Answer from the drawing. Dimensions are ordinates in mm from the lowest x, y and z of the part. A direction names the side the tool comes from. Give positions to 0.01 mm unless a question says otherwise; leave off trailing zeros. Write each loop counter-clockwise with the first axis right and the second up, starting at its lowest first coordinate (ties: lowest second). Pieces come first, ordered by that corner, then holes.
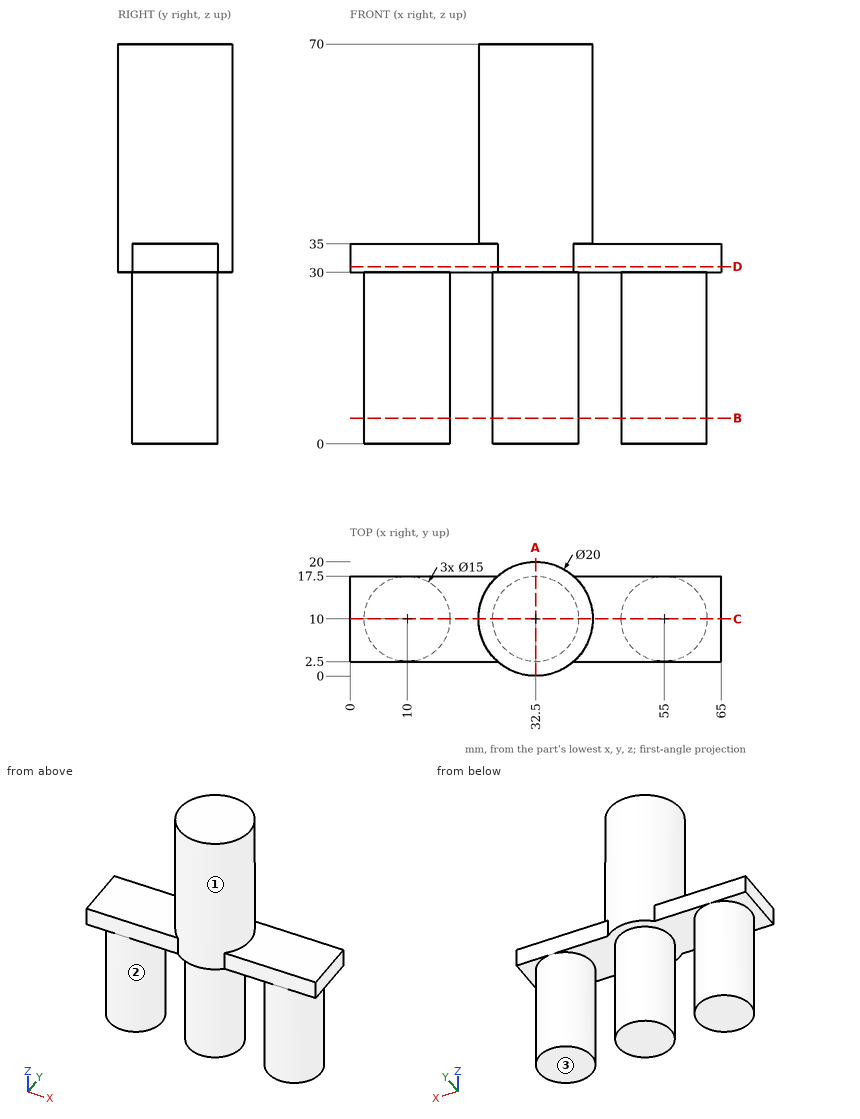
Item 1: A cutting plane is placed at C-C, the plane y = 10. Give the vertices of the cut face in (x, z).
Conclusion:
outline: (0, 30) - (2.5, 30) - (2.5, 0) - (17.5, 0) - (17.5, 30) - (25, 30) - (25, 0) - (40, 0) - (40, 30) - (47.5, 30) - (47.5, 0) - (62.5, 0) - (62.5, 30) - (65, 30) - (65, 35) - (42.5, 35) - (42.5, 70) - (22.5, 70) - (22.5, 35) - (0, 35) - close
Item 2: Each of these flat-tipped pins is pushed along its axis until it touches: P1, Ø5, axis at x = 9.5, y = 10, coming from the +Z side; P2, Ø8, axis at y = 11.5, z = 12, coming from the -X side; P3, Ø3, axis at x = 36, z = 38, coming from the +Y side. Where does it stop, or does it pass through?
Conclusion:
P1: stops at z = 35
P2: stops at x = 2.5
P3: stops at y = 19.8
Item 3: Which of the six approach directions +Z, -Z, +X, -X, +Y, -Y give full straight-line access (tool end or side, diameter ignored) to the marked faces 1, 2 and 3?
Conclusion:
face 1: +Z
face 2: -Z
face 3: -Z, +X, -X, +Y, -Y
Item 4: A cutting plane is placed at A-A, the plane x = 32.5. Give the vertices of the cut face in (y, z), plus the area to 3 significant figures.
Conclusion:
outline: (0, 30) - (2.5, 30) - (2.5, 0) - (17.5, 0) - (17.5, 30) - (20, 30) - (20, 70) - (0, 70) - close
area: 1,250 mm2
Item 5: A cutting plane is placed at B-B, the plane z = 4.5. Give the vertices of the cut face in (x, y).
Conclusion:
outline: circle Ø15 at (10, 10); circle Ø15 at (32.5, 10); circle Ø15 at (55, 10)
Item 6: A cutting plane is placed at D-D, the plane z = 31. Give the vertices of the cut face in (x, y).
Conclusion:
outline: (0, 2.5) - (25.89, 2.5) arc R10 ccw to (39.11, 2.5) - (65, 2.5) - (65, 17.5) - (39.11, 17.5) arc R10 ccw to (25.89, 17.5) - (0, 17.5) - close
Item 7: Consider probe 1 along X at (y, z) = (9.5, 4.5); probe 2 along X at (y, z) = (4.75, 25); probe 3 along Z at (x, y) = (11.5, 14.5). Determine where each line is inside the solid, lowest interval first.
Conclusion:
probe 1: x = 2.52 to 17.48, 25.02 to 39.98, 47.52 to 62.48
probe 2: x = 4.64 to 15.36, 27.14 to 37.86, 49.64 to 60.36
probe 3: z = 0 to 35
